For this review, use the dimensioned drawing (mm, ordinates from the lowest corner) and the shaded views. Coordinates: 2 decimals unless noted, no trailing zeros. Write each loop counter-clockwise with the first axis right and the second up, starting at its lowest first coordinate (ties: lowest second). Pieces come first, ordered by that corner, then holes. Notation, with made-up numbers: M -14,-4 L 45,-4 A22 cw 45,9 Z; hole C 81,6 d4. An arc over 180 degrees is marked long. Return JSON: item names as keys, results as strings. Group by question number.
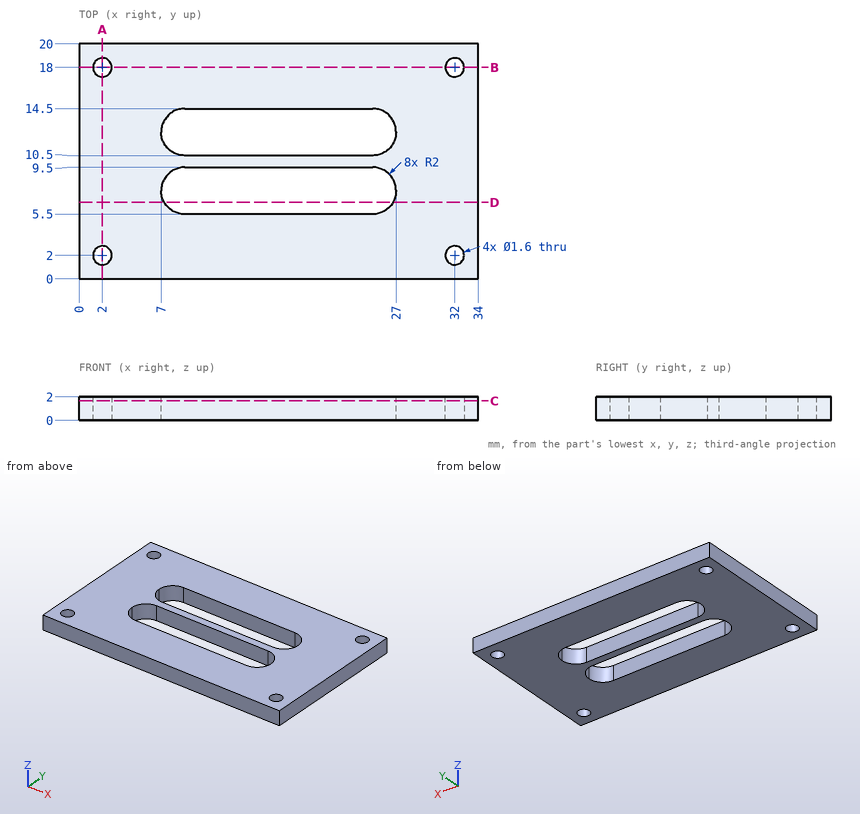
Item 1: Add section D-D (y = 6.5). Write out the cut boundary in (x, z), plus the area to 3 significant figures.
Item 2: Add section B-B (y = 18). Write out the cut boundary in (x, z).
Item 3: For line 1 (Y direction, x = 24, z = 1.35); line 2 (Y direction, x = 2, z = 1.1); line 3 (X direction, y = 2.5, z = 1.3) (1 decimal), list the stretches that pass through material, from the lowest coordinate up.
Item 4: For pin 1 (1 mm diameter, centred on x = 2, y = 2, fed in from -Z), flat-tipped, find the tip position at first contact; note if it passes through.
Item 5: Add section C-C (z = 1.65). Count the separate pieces of the cut face and the enclosed holes in it, plus the area to 3 significant figures.
Item 6: Add section A-A (x = 2). Write out the cut boundary in (y, z).
Geometry check:
{
 "1": {"outline": "M 0,0 L 7.27,0 L 7.27,2 L 0,2 Z; M 26.73,0 L 34,0 L 34,2 L 26.73,2 Z", "area": "29.1 mm^2"},
 "2": {"outline": "M 0,0 L 1.2,0 L 1.2,2 L 0,2 Z; M 2.8,0 L 31.2,0 L 31.2,2 L 2.8,2 Z; M 32.8,0 L 34,0 L 34,2 L 32.8,2 Z"},
 "3": {"line 1": "0 to 5.5, 9.5 to 10.5, 14.5 to 20", "line 2": "0 to 1.2, 2.8 to 17.2, 18.8 to 20", "line 3": "0 to 1.4, 2.6 to 31.4, 32.6 to 34"},
 "4": {"pin 1": "through"},
 "5": {"separate pieces": "1", "enclosed holes": "6", "area": "519 mm^2"},
 "6": {"outline": "M 0,0 L 1.2,0 L 1.2,2 L 0,2 Z; M 2.8,0 L 17.2,0 L 17.2,2 L 2.8,2 Z; M 18.8,0 L 20,0 L 20,2 L 18.8,2 Z"}
}
